Work out the finished part from the listing and answer in its coordinate system (mm). A direction names the side the tool comes from. Coordinates: 2 decimals unless noted, no trailing zeros. Write each loop counter-clockwise with the first axis right and the second up, starting at its lowest first coordinate (ties: lowest second). Pieces come first, ordered by that corner, then holes. Notation, with made-up numbers: (71.25, 15.5) - (120.25, 15.5) arc R20 cw to (120.25, 21.5) - close; hole circle Ø5 at (64, 15). An arc over 180 degrees is marked (long way). Use one line per item in the form item = value. Start each with the question number.
Item 1: For faces 4 (the flat face through (5, 69, 7.5)), 5 (the flat face through (0, 69, 5)), 6 (the flat face through (38, 69, 4)), determine the directions among +Z, -Z, +X, -X, +Y, -Y from which every point of the face is accessible in a straight line to the end or side of a thin tool.
Item 2: A cutting plane is placed at A-A (z = 4). Write down the section's boundary in (x, y), then the cut area to 3 significant figures.
Item 3: A cutting plane is placed at B-B (y = 61). Write down the section's boundary in (x, z), then the cut area to 3 significant figures.
Item 4: A cutting plane is placed at C-C (x = 25.5). Write down the section's boundary in (y, z), then the cut area to 3 significant figures.
Item 5: Determine the mould class of faces 1 (the flat face through (20, 69, 0)), 2 (the flat face through (38, 69, 9)), 3 (the flat face through (2, 69, 4)) for opening direction Z: released by +Z, released by -Z, zero draft, split by the parting line, or undercut.
Item 6: Given pin 1 (5 mm diameter, centred on x = 5, y = 55, fed in from +Z), flat-ended and moving along its own axis, determine where the tip first touches the part or whether it passes through.
Item 7: Consider probe 1 along Z at (x, y) = (34.5, 22.5); probe 2 along X at (y, z) = (130, 5.25); probe 3 along X at (y, z) = (112, 6.75). Determine where each line is inside the solid, lowest interval first.
Autodesk Inventor part; units mm, degrees
ref_plane "YZ Plane" through (0, 0, 0) normal (1, 0, 0) x (0, 1, 0)
ref_plane "XZ Plane" through (0, 0, 0) normal (0, 1, 0) x (-1, 0, 0)
ref_plane "XY Plane" through (0, 0, 0) normal (0, 0, 1) x (1, 0, 0)
sketch "Sketch1" plane through (0, 0, 0) normal (0, 1, 0) x (-1, 0, 0)
  line L0 (0, 0) -> (-40, 0)
  line L1 (-40, 0) -> (-40, -10)
  line L2 (-40, -10) -> (0, -10)
  line L3 (0, -10) -> (0, 0)
  line L4 (0, 0) -> (-40, 0)
  line L5 (-40, 0) -> (-40, -2)
  line L6 (-40, -2) -> (0, -2)
  line L7 (0, -2) -> (0, 0)
  line L8 (0, -10) -> (-2, -10)
  line L9 (-2, -10) -> (-2, 0)
  line L10 (-2, 0) -> (0, 0)
  line L11 (0, 0) -> (0, -10)
  line L12 (-40, -10) -> (-38, -10)
  line L13 (-38, -10) -> (-38, 0)
  line L14 (-38, 0) -> (-40, 0)
  line L15 (-40, 0) -> (-40, -10)
  line L16 (-2, -7.5) -> (-38, -7.5)
  line L17 (-38, -7.5) -> (-38, -5.5)
  line L18 (-38, -5.5) -> (-2, -5.5)
  line L19 (-2, -5.5) -> (-2, -7.5)
  line L20 (-8.5, -10) -> (-31.5, -10)
  line L21 (-31.5, -10) -> (-31.5, -2)
  line L22 (-31.5, -2) -> (-8.5, -2)
  line L23 (-8.5, -2) -> (-8.5, -10)
  point P0 (-38, -10)
  point P1 (-38, -7.5)
  point P2 (-31.5, -7.5)
  point P3 (-31.5, -5.5)
  point P4 (-38, -2)
  point P5 (-2, -2)
  point P6 (-2, -5.5)
  point P7 (-8.5, -5.5)
  point P8 (-8.5, -7.5)
  dimension "d0" = 10
  dimension "d1" = 40
  dimension "d2" = 2
  dimension "d3" = 2
  dimension "d4" = 2
  dimension "d5" = 2
  dimension "d6" = 3.5
  dimension "d7" = 2.5
  dimension "d13" = 6.5
  dimension "d14" = 6.5
extrude "Extrusion1" add sketch "Sketch1" along normal blind 139.7 contours L3 L6 L9 L0 | L9 L6 L13 L0 | L3 L2 L9 L6 | L13 L6 L1 L0 | L13 L2 L1 L6 | L9 L16 L23 L18 | L18 L21 L16 L13
fillet "Fillet1" radius 0.5 2 edges at (31.5, 69.85, -7.5) (31.5, 69.85, -5.5)
fillet "Fillet2" radius 0.5 2 edges at (8.5, 69.85, -5.5) (8.5, 69.85, -7.5)
move or copy body "Rotate1" bodies to move or copy 1 copy no rotation origin (0, 0, 0) rotation axis (0, 1, 0) rotation angle 180 translate (40, 0, 0)
properties part number "lift"
Answer:
q1.face_4 = +Z, +Y, -Y
q1.face_5 = +Z, -Z, -X, +Y, -Y
q1.face_6 = +Y, -Y
q2.outline = (0, 0) - (2, 0) - (2, 139.7) - (0, 139.7) - close; (38, 0) - (40, 0) - (40, 139.7) - (38, 139.7) - close
q2.area = 559 mm²
q3.outline = (0, 0) - (40, 0) - (40, 10) - (38, 10) - (38, 7.5) - (32, 7.5) arc R0.5 ccw to (31.5, 7) - (31.5, 6) arc R0.5 ccw to (32, 5.5) - (38, 5.5) - (38, 2) - (2, 2) - (2, 5.5) - (8, 5.5) arc R0.5 ccw to (8.5, 6) - (8.5, 7) arc R0.5 ccw to (8, 7.5) - (2, 7.5) - (2, 10) - (0, 10) - close
q3.area = 138 mm²
q4.outline = (0, 0) - (139.7, 0) - (139.7, 2) - (0, 2) - close
q4.area = 279 mm²
q5.face_1 = released by -Z
q5.face_2 = zero draft
q5.face_3 = undercut
q6.pin_1 = 7.5
q7.probe_1 = 0 to 2, 5.5 to 7.5
q7.probe_2 = 0 to 2, 38 to 40
q7.probe_3 = 0 to 8.5, 31.5 to 40
